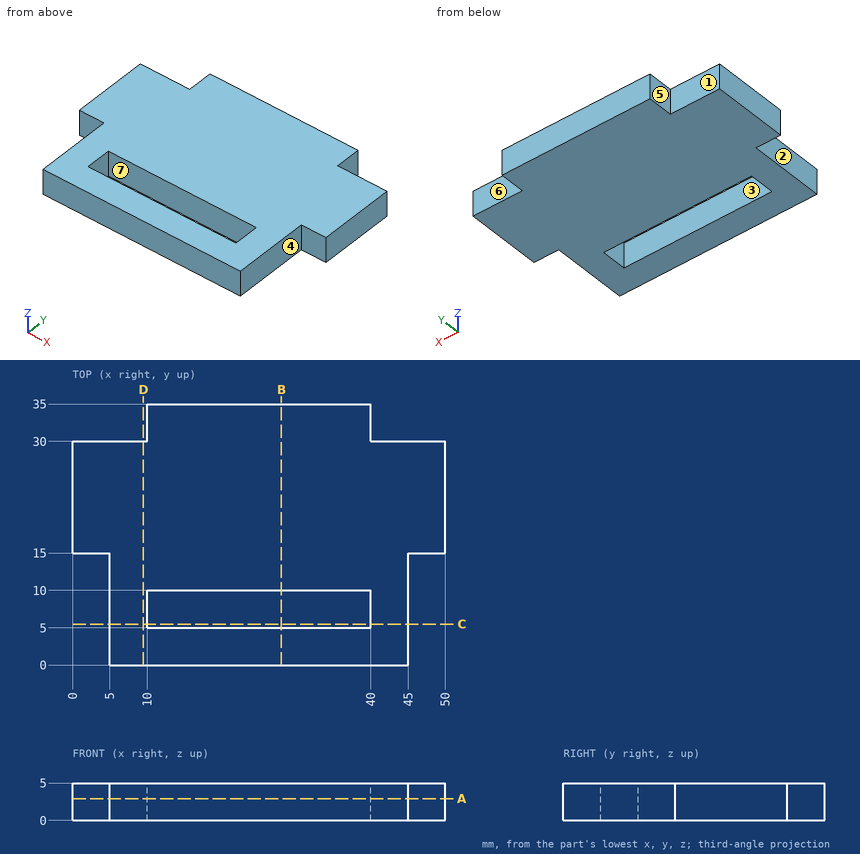
Drawing for the job (mm, zero at the part's lowest x, y, z). A direction names the side the tool comes from. Round coordinates to 2 decimals unless told otherwise and drop trailing zeros. Write each loop counter-clockwise with the first axis right and the second up, starting at its lowest first coordinate (ties: lowest second). Pieces come first, ordered by that corner, then holes. Notation, with made-up numbers: (15, -20.5) - (60, -20.5) arc R14 ccw to (60, -8.5) - close; hole circle Ø1 at (3.25, 89.5). An arc over 180 degrees is marked (long way). Return JSON: item names as keys, results as strings. Group by question number.
Item 1: Band-saw the part on B-B on x = 28. List the corners of the cut face in (y, z).
Item 2: Flat gauge pins, fed straight in: pin 1 Ø2.5 at (x, z) = (1.5, 3) entering from -Y; pin 2 Ø1.5 at (x, z) = (2.5, 3.5) entering from +Y; pin 3 Ø3 at (y, z) = (22, 3) entering from -X; pin 4 Ø2.5 at (y, z) = (33, 2) entering from -X. Where does each tip first touch, or does it go through?
Item 3: Mould opens along X. For the marked faces 5, 6 and 7 say: +X half, -X half, draft (parallel to the pull), parting line (faces both ways), or undercut.
Item 4: Band-saw the part on D-D on x = 9.5. List the corners of the cut face in (y, z).
Item 5: 3-axis set-ups, long thin cutter, end or side, ignore diameter. For the marked faces 1, 2, 3 and 4: which of +Z, -Z, +X, -X, +Y, -Y reach the whole face in a straight line?
Item 6: Probe probe 1 along Y at (x, z) = (32.5, 3.15); probe 2 along X at (y, z) = (9.5, 1.55); probe 3 along X at (y, z) = (10.5, 2.7). List the from-to ranges inside material, lowest first.
Item 7: Band-saw the part on C-C on y = 5.5. List the corners of the cut face in (x, z).
Item 8: Band-saw the part on A-A on z = 2.9. List the corners of the cut face in (x, y).
Resolved:
{
 "1": {"outline": "(0, 0) - (5, 0) - (5, 5) - (0, 5) - close; (10, 0) - (35, 0) - (35, 5) - (10, 5) - close"},
 "2": {"pin 1": "stops at y = 15", "pin 2": "stops at y = 30", "pin 3": "stops at x = 0", "pin 4": "stops at x = 10"},
 "3": {"face 5": "-X half", "face 6": "draft", "face 7": "undercut"},
 "4": {"outline": "(0, 0) - (30, 0) - (30, 5) - (0, 5) - close"},
 "5": {"face 1": "+Z, -Z, -X, +Y", "face 2": "+Z, -Z, -X, -Y", "face 3": "+Z, -Z", "face 4": "+Z, -Z, +X, -Y"},
 "6": {"probe 1": "y = 0 to 5, 10 to 35", "probe 2": "x = 5 to 10, 40 to 45", "probe 3": "x = 5 to 45"},
 "7": {"outline": "(5, 0) - (10, 0) - (10, 5) - (5, 5) - close; (40, 0) - (45, 0) - (45, 5) - (40, 5) - close"},
 "8": {"outline": "(0, 15) - (5, 15) - (5, 0) - (45, 0) - (45, 15) - (50, 15) - (50, 30) - (40, 30) - (40, 35) - (10, 35) - (10, 30) - (0, 30) - close; hole (10, 5) - (40, 5) - (40, 10) - (10, 10) - close"}
}
